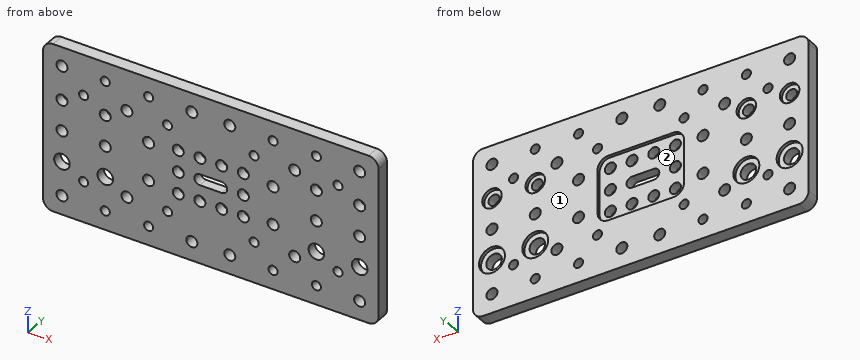
```python
from build123d import *

# Parameters (mm, degrees)
BOSS_EXTRUDE1_DEPTH        = 6
F_5_1_5_1_DIAMETER_HOLE1_D = 5.1
M5X0_8_TAPPED_HOLE1_D      = 4.2
SKETCH6_R                  = 3.6
SKETCH6_R_2                = 2.55
CUT_EXTRUDE1_DEPTH         = 7
SKETCH7_R                  = 6
SKETCH7_R_2                = 4.5
CUT_EXTRUDE2_DEPTH         = 1.5
CUT_EXTRUDE3_DEPTH         = 5.5


with BuildPart() as part:
    # Sketch1 → Boss-Extrude1 (new body)
    with BuildSketch(Plane(origin=(0, 0, 0), x_dir=(1, 0, 0), z_dir=(0, 1, 0))):
        with BuildLine():
            Line((4.64, 0), (150.38, 0))
            ThreePointArc((150.38, 0), (153.660975465, 1.359024535), (155.02, 4.64))
            Line((155.02, 4.64), (155.02, 72.88))
            ThreePointArc((155.02, 72.88), (153.660975465, 76.160975465), (150.38, 77.52))
            Line((150.38, 77.52), (4.64, 77.52))
            ThreePointArc((4.64, 77.52), (1.359024535, 76.160975465), (0, 72.88))
            Line((0, 72.88), (0, 4.64))
            ThreePointArc((0, 4.64), (1.359024535, 1.359024535), (4.64, 0))
        make_face()
    extrude(amount=BOSS_EXTRUDE1_DEPTH)

    # Ø5.1 (5.1) Diameter Hole1 (through all)
    with Locations(Plane(origin=(0, 6, 0), x_dir=(1, 0, 0), z_dir=(0, 1, 0))):
        with Locations((8.755, 68.76), (8.755, 38.76), (28.755, 38.76), (38.755, 58.76), (48.755, 47.515), (68.755, 68.76), (62.485, 48.76), (72.485, 48.76), (62.485, 38.76), (92.535, 38.76), (82.535, 48.76), (92.535, 48.76), (86.265, 68.76), (106.265, 47.515), (116.265, 58.76), (126.265, 38.76), (146.265, 38.76), (146.265, 68.76), (146.265, 8.76), (116.265, 18.76), (106.265, 30.005), (92.535, 28.76), (82.535, 28.76), (86.265, 8.76), (68.755, 8.76), (72.485, 28.76), (62.485, 28.76), (48.755, 30.005), (38.755, 18.76), (8.755, 8.76)):
            Hole(F_5_1_5_1_DIAMETER_HOLE1_D / 2)

    # M5x0.8 Tapped Hole1 (through all)
    with Locations(Plane(origin=(0, 6, 0), x_dir=(1, 0, 0), z_dir=(0, 1, 0))):
        with Locations((18.75, 58.76), (28.755, 68.76), (48.755, 68.76), (57.51, 58.76), (48.755, 8.76), (57.51, 18.76), (18.75, 18.76), (28.755, 8.76), (106.265, 68.76), (97.51, 58.76), (97.51, 18.76), (106.265, 8.76), (126.265, 8.76), (136.27, 18.76), (126.265, 68.76), (136.27, 58.76)):
            Hole(M5X0_8_TAPPED_HOLE1_D / 2)

    # Sketch6 → Cut-Extrude1 (cut, through all)
    with BuildSketch(Plane(origin=(0, 6, 0), x_dir=(1, 0, 0), z_dir=(0, 1, 0))):
        with Locations((8.755, 53.01)):
            Circle(SKETCH6_R)
        with Locations((28.755, 53.01)):
            Circle(SKETCH6_R)
        with Locations((8.755, 24.51)):
            Circle(SKETCH6_R_2)
        with Locations((28.755, 24.51)):
            Circle(SKETCH6_R_2)
        with Locations((126.265, 24.51)):
            Circle(SKETCH6_R_2)
        with Locations((146.265, 24.51)):
            Circle(SKETCH6_R_2)
        with Locations((126.265, 53.01)):
            Circle(SKETCH6_R)
        with Locations((146.265, 53.01)):
            Circle(SKETCH6_R)
    extrude(amount=-CUT_EXTRUDE1_DEPTH, mode=Mode.SUBTRACT)

    # Sketch7 → Cut-Extrude2 (cut)
    with BuildSketch(Plane(origin=(0, 6, 0), x_dir=(1, 0, 0), z_dir=(0, 1, 0))):
        with Locations((8.755, 53.01)):
            Circle(SKETCH7_R)
        with Locations((28.755, 53.01)):
            Circle(SKETCH7_R)
        with Locations((8.755, 24.51)):
            Circle(SKETCH7_R_2)
        with Locations((28.755, 24.51)):
            Circle(SKETCH7_R_2)
        with Locations((126.265, 24.51)):
            Circle(SKETCH7_R_2)
        with Locations((146.265, 24.51)):
            Circle(SKETCH7_R_2)
        with Locations((126.265, 53.01)):
            Circle(SKETCH7_R)
        with Locations((146.265, 53.01)):
            Circle(SKETCH7_R)
        with BuildLine():
            Line((62.475, 53.71), (92.545, 53.71))
            ThreePointArc((92.545, 53.71), (96.038107499, 52.263107499), (97.485, 48.77))
            Line((97.485, 48.77), (97.485, 28.75))
            ThreePointArc((97.485, 28.75), (96.038107499, 25.256892501), (92.545, 23.81))
            Line((92.545, 23.81), (62.475, 23.81))
            ThreePointArc((62.475, 23.81), (58.981892501, 25.256892501), (57.535, 28.75))
            Line((57.535, 28.75), (57.535, 48.77))
            ThreePointArc((57.535, 48.77), (58.981892501, 52.263107499), (62.475, 53.71))
        make_face()
    extrude(amount=-CUT_EXTRUDE2_DEPTH, mode=Mode.SUBTRACT)

    # Sketch8 → Cut-Extrude3 (cut, through all)
    with BuildSketch(Plane(origin=(0, 4.5, 0), x_dir=(1, 0, 0), z_dir=(0, 1, 0))):
        with BuildLine():
            Line((72.485, 41.31), (82.535, 41.31))
            ThreePointArc((82.535, 41.31), (85.085, 38.76), (82.535, 36.21))
            Line((82.535, 36.21), (72.485, 36.21))
            ThreePointArc((72.485, 36.21), (69.935, 38.76), (72.485, 41.31))
        make_face()
    extrude(amount=-CUT_EXTRUDE3_DEPTH, mode=Mode.SUBTRACT)


solid = part.part
```
Check sheet for the modelled part. Datum: model origin and axes. Units: mm. Face numbers are marked on the shaded views. Coordinates: 2 decimals unless noted, no trailing zeros. Loops run counter-clockwise (first coordinate to the right, second up) from the corner with the lowest first, then second, coordinate; pieces in that order, holes last. Notation, with made-up numbers: M -38,-13 L 18,-13 A26 cw 18,8 Z; hole C 10.25,25 d2. An arc over 180 degrees is marked long. Answer as a JSON object with one key per item and string values.
1. Scan lines: L1, parallel to Z at x = 57.51, y = 2.6; L2, parallel to Z at x = 107.5, y = 2.7; L3, parallel to Z at x = 89, y = 5.35. Record each from-to range of solid material in increasing order. Write a range as from..to.
Outcome:
{"L1": "-77.52..-60.86, -56.66..-20.86, -16.66..0", "L2": "-77.52..-70.46, -67.06..-49.75, -45.28..-32.24, -27.77..-10.46, -7.06..0", "L3": "-77.52..-53.71, -23.81..0"}
2. Sectioned sample at B-B on z = -38.76. Count the separate pieces of the cut face and the enclosed holes in it, and give its area (3 significant figures).
Outcome:
{"separate pieces": "8", "enclosed holes": "0", "area": "634 mm²"}
3. Sectioned sample at A-A on x = 136.27. Record the cut outline in (y, z).
Outcome:
{"outline": "M 0,-77.52 L 6,-77.52 L 6,-60.86 L 0,-60.86 Z; M 0,-56.66 L 6,-56.66 L 6,-20.86 L 0,-20.86 Z; M 0,-16.66 L 6,-16.66 L 6,0 L 0,0 Z"}
4. Release check for a two-part mould opening along X. For the marked faces 1 and 2 record: pulls with the +X half, pulls with the -X half, needs draft (parallel to the pull), parting line crosses it, or undercut.
Outcome:
{"face 1": "needs draft", "face 2": "undercut"}
5. Depth check by flat-ended pin: P1, Ø8, axis at x = 146.265, z = -24.51, coming from the +Y side. Enter the tip coordinate at first touch or a pass-through.
Outcome:
{"P1": "y = 4.5"}
